Source: CAD feature listing. Evaluate the final solid. Frame: model axes, mm. Round coordinates to 2 decimals unless told otherwise and drop trailing zeros. Loops run counter-clockwise (first coordinate to the right, second up) from the corner with the lowest first, then second, coordinate; pieces in that order, holes last. Notation, with made-up numbers: M -1.75,-24 L 26.25,-24 A25 cw 26.25,-11 Z; hole C 56.25,85 d11. An arc over 180 degrees is marked long. Answer as CSV lines item,"result". Start each with the question number.
```python
from build123d import *
from build123d.topology import SkipClean

# Parameters (mm, degrees)
SKETCH1_R           = 6.5
SKETCH1_R_2         = 4.5
BOSS_EXTRUDE1_DEPTH = 0.8
SKETCH2_R           = 2
BOSS_EXTRUDE2_DEPTH = 0.8
CUT_EXTRUDE1_START  = -0.8
CUT_EXTRUDE1_DEPTH  = 0.8
SKETCH4_R           = 1
CUT_EXTRUDE2_DEPTH  = 0.8
FILLET1_R           = 3


with BuildPart() as part:
    # Sketch1 → Boss-Extrude1 (new body)
    with BuildSketch(Plane.XY):
        Circle(SKETCH1_R)
        Circle(SKETCH1_R_2, mode=Mode.SUBTRACT)
    extrude(amount=BOSS_EXTRUDE1_DEPTH)

    # Sketch2 → Boss-Extrude2 (add)
    with BuildSketch(Plane.XY.offset(0.8)):
        with Locations((-4.596194078, -4.596194078)):
            Circle(SKETCH2_R)
        with Locations((4.596194078, -4.596194078)):
            Circle(SKETCH2_R)
    extrude(amount=-BOSS_EXTRUDE2_DEPTH)

    # Sketch3 → Cut-Extrude1 (cut)
    with SkipClean():  # the faces are left unmerged after this step: merging them gives an invalid solid
        with BuildSketch(Plane.XY.offset(0.8).offset(CUT_EXTRUDE1_START)):
            with BuildLine():
                ThreePointArc((-2.981245674, -5.775999847), (-2.602155556, -4.441887978), (-3.181980515, -3.181980515))
                ThreePointArc((-3.181980515, -3.181980515), (0, -4.5), (3.181980515, -3.181980515))
                ThreePointArc((3.181980515, -3.181980515), (2.602155556, -4.441887978), (2.981245674, -5.775999847))
                ThreePointArc((2.981245674, -5.775999847), (0, -6.5), (-2.981245674, -5.775999847))
            make_face()
        extrude(amount=CUT_EXTRUDE1_DEPTH, mode=Mode.SUBTRACT)

    # Sketch4 → Cut-Extrude2 (cut)
    with SkipClean():  # the faces are left unmerged after this step: merging them gives an invalid solid
        with BuildSketch(Plane.XY.offset(0.8)):
            with Locations((-4.596194078, -4.596194078)):
                Circle(SKETCH4_R)
            with Locations((4.596194078, -4.596194078)):
                Circle(SKETCH4_R)
        extrude(amount=-CUT_EXTRUDE2_DEPTH, mode=Mode.SUBTRACT)

    # Fillet1
    fillet1_edges = [part.edges().sort_by_distance(p)[0] for p in [
        (-5.775999847, -2.981245674, 0.4),
        (5.775999847, -2.981245674, 0.4),
    ]]
    fillet(fillet1_edges, radius=FILLET1_R)


solid = part.part
```
1) Section B-B, the plane x = 2.75. Return loops of the section in (y, z), and give its area (3 significant figures).
2) Mould query, pull axis X, two halves, no side actions, for faces 1 (the cylindrical face through (0.1, 4.5, 0.4)), 2 (the cylindrical face through (0.168, 6.498, 0.394)), 3 (the flat face through (-4.5, -1.4, 0.8)), 4 (the cylindrical face through (5.55, -4.3, 0.41)). Classes: pulls with the +X half, pulls with the -X half, needs draft (parallel to the pull), parting line crosses it, or undercut.
3) Ray query, line 1 along X through (y, z) = (-4.25, 0.7); line 2 along X through (y, z) = (-5.5, 0.4); line 3 along X through (y, z) = (0, 0.4). Return the intervals inside material, ascending.
4) Section C-C, the plane z = 0.25. Give the number of separate pieces and of enclosed holes in the cut face, and give its area (3 significant figures).
5) Section A-A, the plane y = 0. Return loops of the section in (x, z), and give its area (3 significant figures).
6) Section D-D, the plane x = 0. Return loops of the section in (y, z).
Findings below:
1,outline,"M -5.37,0 L -3.83,0 L -3.83,0.8 L -5.37,0.8 Z; M 3.56,0 L 5.89,0 L 5.89,0.8 L 3.56,0.8 Z"
1,area,"3.09 mm²"
2,face 1,"undercut"
2,face 2,"parting line crosses it"
2,face 3,"needs draft"
2,face 4,"undercut"
3,line 1,"-6.57 to -5.53, -3.66 to -2.63, 2.63 to 3.66, 5.53 to 6.57"
3,line 2,"-6.38 to -5.02, -4.17 to -2.81, 2.81 to 4.17, 5.02 to 6.38"
3,line 3,"-6.5 to -4.5, 4.5 to 6.5"
4,separate pieces,"1"
4,enclosed holes,"2"
4,area,"65.4 mm²"
5,outline,"M -6.5,0 L -4.5,0 L -4.5,0.8 L -6.5,0.8 Z; M 4.5,0 L 6.5,0 L 6.5,0.8 L 4.5,0.8 Z"
5,area,"3.20 mm²"
6,outline,"M 4.5,0 L 6.5,0 L 6.5,0.8 L 4.5,0.8 Z"
